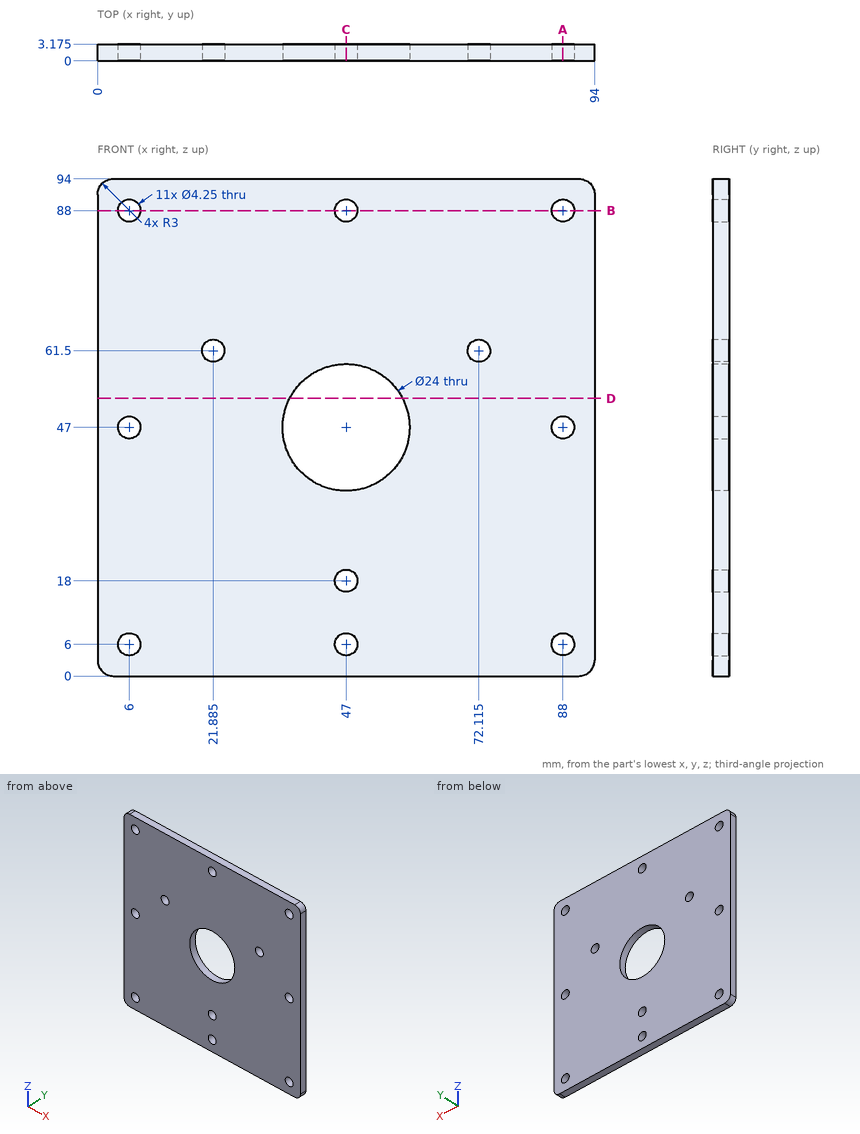
Geometry check sheet. Reference: drawing and pictorial views, mm from the part's lowest x, y, z. Round coordinates to 2 decimals unless told otherwise and drop trailing zeros. Order: outer loops, then holes, each group sorted by start corner. A loop starts at its lowest first (then second) coordinate and runs counter-clockwise, first axis right, second up. Notation, with made-up numbers: M 4.25,36 L 24.25,36 A22 ccw 24.25,71 Z; hole C 53.25,-24.75 d8. An arc over 180 degrees is marked long. Answer in a Markdown table with one row per item.
(1) Scan lines: probe 1 along X at (y, z) = (0.85, 6) (1 decimal); probe 2 along X at (y, z) = (1.1, 61.5). Record each from-to range of solid material in increasing order. Write a range as from..to.
Responses:
| item | result |
|---|---|
| probe 1 | x = 0..3.9, 8.1..44.9, 49.1..85.9, 90.1..94 |
| probe 2 | x = 0..19.76, 24.01..69.99, 74.24..94 |
(2) Sectioned sample at C-C, the plane x = 47. Record the cut outline in (y, z) (1 decimal), and give its area (3 significant figures).
Responses:
| item | result |
|---|---|
| outline | M 0,0 L 3.2,0 L 3.2,3.9 L 0,3.9 Z; M 0,8.1 L 3.2,8.1 L 3.2,15.9 L 0,15.9 Z; M 0,20.1 L 3.2,20.1 L 3.2,35 L 0,35 Z; M 0,59 L 3.2,59 L 3.2,85.9 L 0,85.9 Z; M 0,90.1 L 3.2,90.1 L 3.2,94 L 0,94 Z |
| area | 182 mm² |
(3) Sectioned sample at B-B, the plane z = 88. Record the cut outline in (x, y) (1 decimal), and give its area (3 significant figures).
Responses:
| item | result |
|---|---|
| outline | M 0,0 L 3.9,0 L 3.9,3.2 L 0,3.2 Z; M 8.1,0 L 44.9,0 L 44.9,3.2 L 8.1,3.2 Z; M 49.1,0 L 85.9,0 L 85.9,3.2 L 49.1,3.2 Z; M 90.1,0 L 94,0 L 94,3.2 L 90.1,3.2 Z |
| area | 258 mm² |
(4) Sectioned sample at A-A, the plane x = 88. Record the cut outline in (y, z) (1 decimal).
Responses:
| item | result |
|---|---|
| outline | M 0,0 L 3.2,0 L 3.2,3.9 L 0,3.9 Z; M 0,8.1 L 3.2,8.1 L 3.2,44.9 L 0,44.9 Z; M 0,49.1 L 3.2,49.1 L 3.2,85.9 L 0,85.9 Z; M 0,90.1 L 3.2,90.1 L 3.2,94 L 0,94 Z |
(5) Sectioned sample at D-D, the plane z = 52.5. Record the cut outline in (x, y) (1 decimal), and give its area (3 significant figures).
Responses:
| item | result |
|---|---|
| outline | M 0,0 L 36.3,0 L 36.3,3.2 L 0,3.2 Z; M 57.7,0 L 94,0 L 94,3.2 L 57.7,3.2 Z |
| area | 231 mm² |
(6) Go/stop test with flat-tipped pins: P1, Ø5, axis at x = 72.11, z = 61.5, coming from the +Y side (3 decimals); P2, Ø2.5, axis at x = 88, z = 47, coming from the -Y side. Record where each tip stops, or that it passes through.
Responses:
| item | result |
|---|---|
| P1 | stops at y = 3.175 |
| P2 | passes through |
